Autodesk Inventor part; units mm, degrees
ref_plane "YZ Plane" through (0, 0, 0) normal (1, 0, 0) x (0, 1, 0)
ref_plane "XZ Plane" through (0, 0, 0) normal (0, 1, 0) x (-1, 0, 0)
ref_plane "XY Plane" through (0, 0, 0) normal (0, 0, 1) x (1, 0, 0)
sketch "Sketch1" plane through (0, 0, 0) normal (0, 0, 1) x (1, 0, 0)
  circle A0 centre (0, 0) radius 15.875
  dimension "d0" = 31.75
extrude "mainBody" add sketch "Sketch1" along normal blind 86.5188
sketch "Sketch14" plane through (0, 0, 86.5188) normal (0, 0, 1) x (1, 0, 0)
  circle A0 centre (0, 0) radius 15.875
  circle A1 centre (0, 0) radius 10.4648
  dimension "d43" = 20.9296
extrude "mainTube" cut sketch "Sketch14" against normal blind 177.8 contours A1
sketch "Sketch15" plane through (0, 0, 86.5188) normal (0, 0, 1) x (1, 0, 0)
  circle A0 centre (0, 0) radius 10.4648
  circle A1 centre (0, 0) radius 15.875
  circle A2 centre (0, 0) radius 13.335
  dimension "d47" = 26.67
extrude "mainSocket1" cut sketch "Sketch15" against normal blind 25.4 contours A2
sketch "Sketch16" plane through (0, 0, 0) normal (0, 0, -1) x (-1, 0, 0)
  circle A0 centre (0, 0) radius 10.4648
  circle A1 centre (0, 0) radius 15.875
  circle A2 centre (0, 0) radius 13.335
  dimension "d51" = 26.67
extrude "mainSocket2" cut sketch "Sketch16" against normal blind 25.4 contours A2
properties part number "0pvc_T_0.75" material "PVC-Piping"
Verification items for the finished model (mm, model axes). A direction names the side the tool comes from. Round coordinates to 2 decimals unless told otherwise and drop trailing zeros. Loops run counter-clockwise (first coordinate to the right, second up) from the corner with the lowest first, then second, coordinate; pieces in that order, holes last. Notation, with made-up numbers: (57.25, 25.25) - (73.25, 25.25) arc R12 ccw to (73.25, 33.25) - close; hole circle Ø1 at (16.5, 78.25). An arc over 180 degrees is marked (long way). Write item = value, one per line.
Q1. Sectioned sample at A-A on x = 0. Record the boundary of the cut face in (y, z) (3 decimals), plus the area to 3 significant figures.
Here are the results:
outline = (-15.875, 0) - (-13.335, 0) - (-13.335, 25.4) - (-10.465, 25.4) - (-10.465, 61.119) - (-13.335, 61.119) - (-13.335, 86.519) - (-15.875, 86.519) - close; (10.465, 25.4) - (13.335, 25.4) - (13.335, 0) - (15.875, 0) - (15.875, 86.519) - (13.335, 86.519) - (13.335, 61.119) - (10.465, 61.119) - close
area = 645 mm^2
Q2. Sectioned sample at D-D on z = 18. Record the boundary of the cut face in (x, y) (3 decimals).
Here are the results:
outline = circle Ø31.75 at (0, 0); hole circle Ø26.67 at (0, 0)
Q3. Mould release check, pull along Y, two halves, no side actions. Record for faces 4 (the cylindrical face through (-3.441, 15.497, 42.654)), 5 (the cylindrical face through (1.74, 13.22, 12.52)), 6 (the flat face through (-4, 13, 0)): +Y half, -Y half, draft (parallel to the pull), parting line (faces both ways), or undercut.
Here are the results:
face_4 = parting line
face_5 = undercut
face_6 = draft
Q4. Depth check by flat-ended pin: pin 1 (2 mm diameter, centred on y = 7.5, z = 35.5, fed in from -X); pin 2 (1 mm diameter, centred on x = -6.5, z = 10.5, fed in from -Y); pin 3 (4 mm diameter, centred on y = 3.5, z = 28, fed in from -X). Enter the tip coordinate at first touch or a pass-through.
Here are the results:
pin_1 = -14.48
pin_2 = -14.7
pin_3 = -15.8
Q5. Material ranges on L1, parallel to Y at x = 0, z = 17 (3 decimals); L2, parallel to X at y = 2.5, z = 56.5; L3, parallel to X at y = 4, z = 46, recorded low to high.
Here are the results:
L1 = -15.875 to -13.335, 13.335 to 15.875
L2 = -15.68 to -10.16, 10.16 to 15.68
L3 = -15.36 to -9.67, 9.67 to 15.36
Q6. Tool access check on faces 1 (the cylindrical face through (-1.74, 13.22, 74)), 2 (the cylindrical face through (-2.269, -10.216, 43.509)), 3 (the flat face through (8, -7, 25.4)). Record the directions out of +Z, -Z, +X, -X, +Y, -Y that give a thin tool (end or side, any length) a straight path to the whole face; none if there is none.
Here are the results:
face_1 = +Z
face_2 = +Z, -Z
face_3 = -Z
Q7. Sectioned sample at C-C on z = 33. Record the boundary of the cut face in (x, y) (3 decimals).
Here are the results:
outline = circle Ø31.75 at (0, 0); hole circle Ø20.93 at (0, 0)
